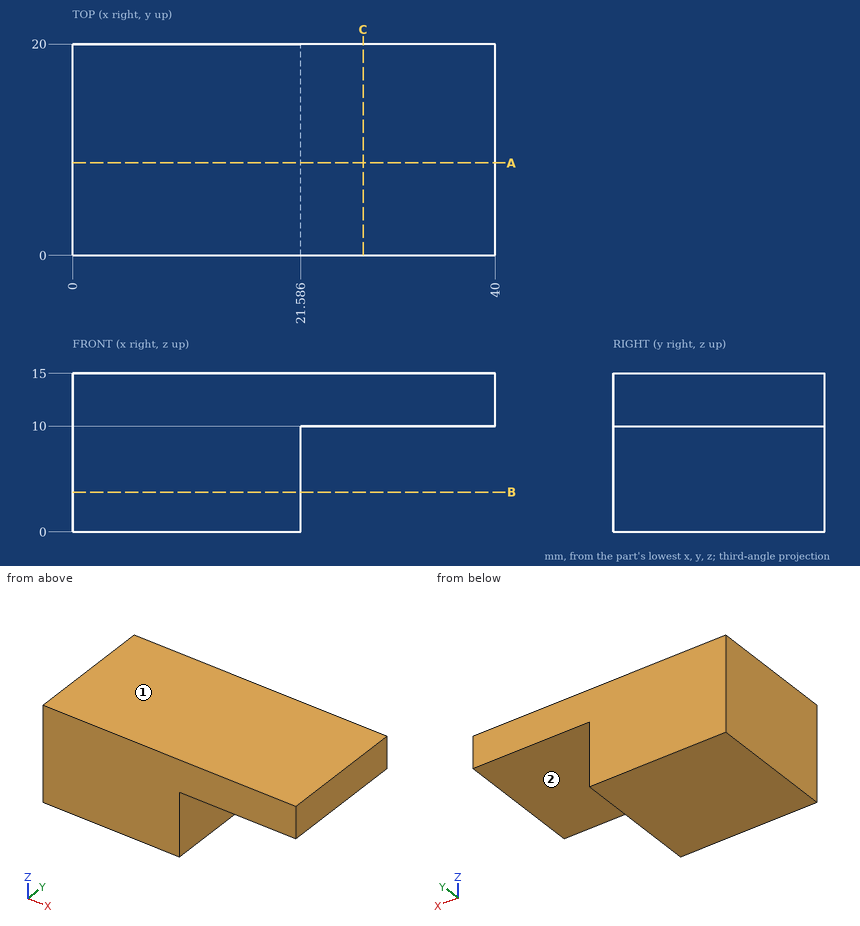
Here's the drawing with two shaded views (mm, measured from the low corner). I have some questions. A direction names the side the tool comes from. Give positions to 0.01 mm unless a question says otherwise; leave off trailing zeros. Loops run counter-clockwise (first coordinate to the right, second up) from the corner with the lowest first, then second, coordinate; pieces in that order, holes last. Notation, with made-up numbers: (-31, 60.5) - (21, 60.5) arc R16 ccw to (21, 83.5) - close; hole circle Ø7 at (-2, 73.5). An arc over 180 degrees is marked (long way). One line per item, written item: value.
(1) If we section it at B-B, the plane z = 3.75: List the corners of the cut face in (x, y) for me, plus the area to 3 significant figures.
Verdict:
outline: (0, 0) - (21.59, 0) - (21.59, 20) - (0, 20) - close
area: 432 mm^2
(2) On a 3-axis mill with a long thin cutter (end or side, diameter ignored), from which of +Z, -Z, +X, -X, +Y, -Y can I reach the whole of each face in a straight line? I mean the marked faces 1 and 2. Say none if no direction works.
Verdict:
face 1: +Z, +X, -X, +Y, -Y
face 2: -Z, +X, +Y, -Y
(3) If we section it at A-A, the plane y = 8.75: List the corners of the cut face in (x, z) for me, plus the area to 3 significant figures.
Verdict:
outline: (0, 0) - (21.59, 0) - (21.59, 10) - (40, 10) - (40, 15) - (0, 15) - close
area: 416 mm^2
(4) If we section it at C-C, the plane x = 27.5: List the corners of the cut face in (y, z) for me, plus the area to 3 significant figures.
Verdict:
outline: (0, 10) - (20, 10) - (20, 15) - (0, 15) - close
area: 100 mm^2
(5) I'm going to push a flat-ended pin straight in: pin 1 (1 mm diameter, centred on y = 16, z = 4, fed in from +X). Where does the tip first touch, or does it pass through?
Verdict:
pin 1: x = 21.59
(6) I need wall thicknesses on line 1 along Z through (x, y) = (38.5, 14); line 2 along X through (y, z) = (12.75, 5.25). Which ranges of each line are inside material? Lowest first, please.
Verdict:
line 1: 10 to 15
line 2: 0 to 21.59
